from build123d import *

# Parameters (mm, degrees)
EXTRUDE_1_DEPTH          = 11.5
CUT_EXTRUDE_1_DEPTH      = 25.129857024
CUT_EXTRUDE_1_DEPTH_BACK = 25.129857024
SKETCH_2_R               = 4.5


with BuildPart() as part:
    # 草图1 → 凸台-拉伸1 (new, symmetric)
    with BuildSketch(Plane(origin=(0, 0, 0), x_dir=(1, 0, 0), z_dir=(0, 1, 0))):
        with BuildLine():
            Line((-11, -15), (11, -15))
            ThreePointArc((11, -15), (13.828427125, -13.828427125), (15, -11))
            Line((15, -11), (15, 11))
            ThreePointArc((15, 11), (13.828427125, 13.828427125), (11, 15))
            Line((11, 15), (-11, 15))
            ThreePointArc((-11, 15), (-13.828427125, 13.828427125), (-15, 11))
            Line((-15, 11), (-15, -11))
            ThreePointArc((-15, -11), (-13.828427125, -13.828427125), (-11, -15))
        make_face()
        with BuildLine():
            Line((-11, -13), (11, -13))
            ThreePointArc((11, -13), (12.414213562, -12.414213562), (13, -11))
            Line((13, -11), (13, 11))
            ThreePointArc((13, 11), (12.414213562, 12.414213562), (11, 13))
            Line((11, 13), (-11, 13))
            ThreePointArc((-11, 13), (-12.414213562, 12.414213562), (-13, 11))
            Line((-13, 11), (-13, -11))
            ThreePointArc((-13, -11), (-12.414213562, -12.414213562), (-11, -13))
        make_face(mode=Mode.SUBTRACT)
    extrude(amount=EXTRUDE_1_DEPTH, both=True)

    # 草图2 → 切除-拉伸1 (cut, two sides: drawn at the far end of the back side and taken through both)
    with BuildSketch(Plane(origin=(0, 0, 0), x_dir=(0, 0, -1), z_dir=(1, 0, 0)).offset(-CUT_EXTRUDE_1_DEPTH_BACK)):
        with Locations((0, 14.5)):
            Circle(SKETCH_2_R)
    extrude(amount=CUT_EXTRUDE_1_DEPTH + CUT_EXTRUDE_1_DEPTH_BACK, mode=Mode.SUBTRACT)


solid = part.part
For this review, take the finished solid that the model builds, in its own axes (mm). A direction names the side the tool comes from. Round coordinates to 2 decimals unless told otherwise and drop trailing zeros. Write each loop counter-clockwise with the first axis right and the second up, starting at its lowest first coordinate (ties: lowest second). Pieces come first, ordered by that corner, then holes. Notation, with made-up numbers: M 53,-38.75 L 68,-38.75 A12 cw 68,-15.75 Z; hole C 42.25,-10 d9. An arc over 180 degrees is marked long. Write item = value, one per line. Start each with the question number.
(1) The part is to be moulded in two halves that separate along Z. For faces 1 (the face through (-15, 0, 0)), 2 (the face through (13, 0, 0)), 3 (the face through (0, 0, -13)), 4 (the face through (13.797, 0.161, 13.859)), say which applies: +Z half, -Z half, draft (parallel to the pull), parting line (faces both ways), or undercut.
(2) For faces 5 (the face through (-13.859, 0.161, 13.797)), 6 (the face through (0, 0, 13)), list the 3-axis set-ups (+Z, -Z, +X, -X, +Y, -Y) from which the entire face can be reached by the end or side of a thin tool; tool diameter is ignored.
(3) We need section A-A (x = -6.5). Give the boundary of the cut face in (y, z).
(4) We need section B-B (z = -7). Give the boundary of the cut face in (x, y), then the cut area to 3 significant figures.
(5) We need section C-C (y = 1.5). Give the boundary of the cut face in (x, z).
(6) For line 1 along Z through (x, y) = (6, -8); line 2 along Z through (x, y) = (12, 8), list the stretches that pass through material, from the lowest coordinate up.
Results found:
q1.face_1 = draft
q1.face_2 = undercut
q1.face_3 = undercut
q1.face_4 = +Z half
q2.face_5 = +Z, -X, +Y, -Y
q2.face_6 = +Y, -Y
q3.outline = M -11.5,-15 L 11.5,-15 L 11.5,-13 L -11.5,-13 Z; M -11.5,13 L 11.5,13 L 11.5,15 L -11.5,15 Z
q4.outline = M -15,-11.5 L -13,-11.5 L -13,11.5 L -15,11.5 Z; M 13,-11.5 L 15,-11.5 L 15,11.5 L 13,11.5 Z
q4.area = 92.0 mm²
q5.outline = M -15,-11 A4 ccw -11,-15 L 11,-15 A4 ccw 15,-11 L 15,11 A4 ccw 11,15 L -11,15 A4 ccw -15,11 Z; hole M -13,-11 A2 ccw -11,-13 L 11,-13 A2 ccw 13,-11 L 13,11 A2 ccw 11,13 L -11,13 A2 ccw -13,11 Z
q6.line_1 = -15 to -13, 13 to 15
q6.line_2 = -14.87 to -12.73, 12.73 to 14.87
